```python
from build123d import *

# Parameters (mm, degrees)
SKICA1_W                 = 30
SKICA1_H                 = 150
P_IDAT_VYSUNUT_M1_DEPTH  = 5
ZAOBLIT1_R               = 10
SKICA2_W                 = 13
SKICA2_H                 = 25
ODEBRAT_VYSUNUT_M1_DEPTH = 6
SKICA3_R                 = 0.5
ODEBRAT_VYSUNUT_M2_DEPTH = 6
ODEBRAT_VYSUNUT_M3_DEPTH = 2
SKICA5_R                 = 0.5
ODEBRAT_VYSUNUT_M4_DEPTH = 4
SKICA6_R                 = 3.75
ODEBRAT_VYSUNUT_M5_DEPTH = 4
SKICA7_W                 = 7.5
SKICA7_H                 = 8
ODEBRAT_VYSUNUT_M6_DEPTH = 6


with BuildPart() as part:
    # Skica1 → Přidat vysunutím1 (new body)
    with BuildSketch(Plane.XY):
        with Locations((15, 75)):
            Rectangle(SKICA1_W, SKICA1_H)
    extrude(amount=P_IDAT_VYSUNUT_M1_DEPTH)

    # Zaoblit1
    zaoblit1_edges = [part.edges().sort_by_distance(p)[0] for p in [
        (0, 150, 2.5),
        (30, 150, 2.5),
        (30, 0, 2.5),
        (0, 0, 2.5),
    ]]
    fillet(zaoblit1_edges, radius=ZAOBLIT1_R)

    # Skica2 → Odebrat vysunutím1 (cut, through all)
    with BuildSketch(Plane.XY.offset(5)):
        with Locations((15, 127.5)):
            Rectangle(SKICA2_W, SKICA2_H)
    extrude(amount=-ODEBRAT_VYSUNUT_M1_DEPTH, mode=Mode.SUBTRACT)

    # Skica3 → Odebrat vysunutím2 (cut, through all)
    with BuildSketch(Plane.XY.offset(5)):
        with Locations((15, 141.5)):
            Circle(SKICA3_R)
        with Locations((15, 113.5)):
            Circle(SKICA3_R)
    extrude(amount=-ODEBRAT_VYSUNUT_M2_DEPTH, mode=Mode.SUBTRACT)

    # Skica4 → Odebrat vysunutím3 (cut)
    with BuildSketch(Plane.XY.offset(5)):
        Polygon((18.40625, 20), (11.59375, 20), (13, 5), (17, 5), align=None)
        Polygon((18.5, 21), (11.5, 21), (11.59375, 20), (18.40625, 20), align=None)
        Polygon((11.59375, 20), (11.5, 21), (11.772727273, 24), (8, 24), (8, 20), align=None)
        Polygon((11.772727273, 24), (11.5, 21), (18.5, 21), (18.227272727, 24), align=None)
        Polygon((18.227272727, 24), (18.5, 21), (18.40625, 20), (22, 20), (22, 24), align=None)
        with BuildLine():
            ThreePointArc((22, 24), (24, 22), (22, 20))
            Line((22, 20), (22, 24))
        make_face()
        with BuildLine():
            Line((8, 24), (8, 20))
            ThreePointArc((8, 20), (6, 22), (8, 24))
        make_face()
        Polygon((13.5, 43), (11.772727273, 24), (18.227272727, 24), (16.5, 43), align=None)
    extrude(amount=-ODEBRAT_VYSUNUT_M3_DEPTH, mode=Mode.SUBTRACT)

    # Skica5 → Odebrat vysunutím4 (cut, through all)
    with BuildSketch(Plane.XY.offset(3)):
        with Locations((15, 36.2)):
            Circle(SKICA5_R)
        with Locations((15, 9.7)):
            Circle(SKICA5_R)
    extrude(amount=-ODEBRAT_VYSUNUT_M4_DEPTH, mode=Mode.SUBTRACT)

    # Skica6 → Odebrat vysunutím5 (cut, through all)
    with BuildSketch(Plane.XY.offset(3)):
        with Locations((15, 22)):
            Circle(SKICA6_R)
    extrude(amount=-ODEBRAT_VYSUNUT_M5_DEPTH, mode=Mode.SUBTRACT)

    # Skica7 → Odebrat vysunutím6 (cut, through all)
    with BuildSketch(Plane.XY.offset(5)):
        with Locations((7.84375, 16)):
            Rectangle(SKICA7_W, SKICA7_H)
    extrude(amount=-ODEBRAT_VYSUNUT_M6_DEPTH, mode=Mode.SUBTRACT)


solid = part.part
```
Check sheet for the modelled part. Datum: model origin and axes. Units: mm. A direction names the side the tool comes from. Coordinates: 2 decimals unless noted, no trailing zeros. Write each loop counter-clockwise with the first axis right and the second up, starting at its lowest first coordinate (ties: lowest second). Pieces come first, ordered by that corner, then holes. Notation, with made-up numbers: M -33,18 L -27,18 A17 ccw -27,28 Z; hole C -5,-27.75 d3. An arc over 180 degrees is marked long. Write item = value, one per line. Start each with the question number.
1. Mould release check, pull along Y, two halves, no side actions. Record for faces 1 (the flat face through (30, 74, 2)), 2 (the flat face through (8, 12, 3)), 3 (the flat face through (21.5, 127, 3)), 4 (the cylindrical face through (2.85, 3.01, 2.54)): pulls with the +Y half, pulls with the -Y half, needs draft (parallel to the pull), parting line crosses it, or undercut.
2. Sectioned sample at B-B (y = 117). Record the cut outline in (x, z), then the cut area to 3 significant figures.
3. Tool access check on faces 5 (the flat face through (11.594, 16, 3)), 6 (the flat face through (13, 25.5, 3)), 7 (the flat face through (0, 74, 2)). Record the directions out of +Z, -Z, +X, -X, +Y, -Y that give a thin tool (end or side, any length) a straight path to the whole face; none if there is none.
4. Sectioned sample at A-A (y = 22). Record the cut outline in (x, z).
5. Thickness scan on probe 1 along Y at (x, z) = (10.25, 1.6); probe 2 along Y at (x, z) = (14, 0.4); probe 3 along X at (y, z) = (36.2, 1.5). Record the ranges inside material, lowest first.
6. Go/stop test with flat-tipped pins: pin 1 (6 mm diameter, centred on x = 13, y = 120.5, fed in from -Z); pin 2 (1 mm diameter, centred on x = 19, y = 17.5, fed in from -Z); pin 3 (1.5 mm diameter, centred on x = 8, z = 3.5, fed in from -Y). Record where each tip stops, or that it passes through.
The answers:
q1.face_1 = needs draft
q1.face_2 = undercut
q1.face_3 = undercut
q1.face_4 = pulls with the -Y half
q2.outline = M 0,0 L 8.5,0 L 8.5,5 L 0,5 Z; M 21.5,0 L 30,0 L 30,5 L 21.5,5 Z
q2.area = 85.0 mm²
q3.face_5 = +Z, -Z
q3.face_6 = +Z
q3.face_7 = +Z, -Z, -X, +Y, -Y
q4.outline = M 0,0 L 11.25,0 L 11.25,3 L 6,3 L 6,5 L 0,5 Z; M 18.75,0 L 30,0 L 30,5 L 24,5 L 24,3 L 18.75,3 Z
q5.probe_1 = 0 to 12, 20 to 115, 140 to 150
q5.probe_2 = 0 to 18.39, 25.61 to 115, 140 to 150
q5.probe_3 = 0 to 14.5, 15.5 to 30
q6.pin_1 = through
q6.pin_2 = 0
q6.pin_3 = 0.08
